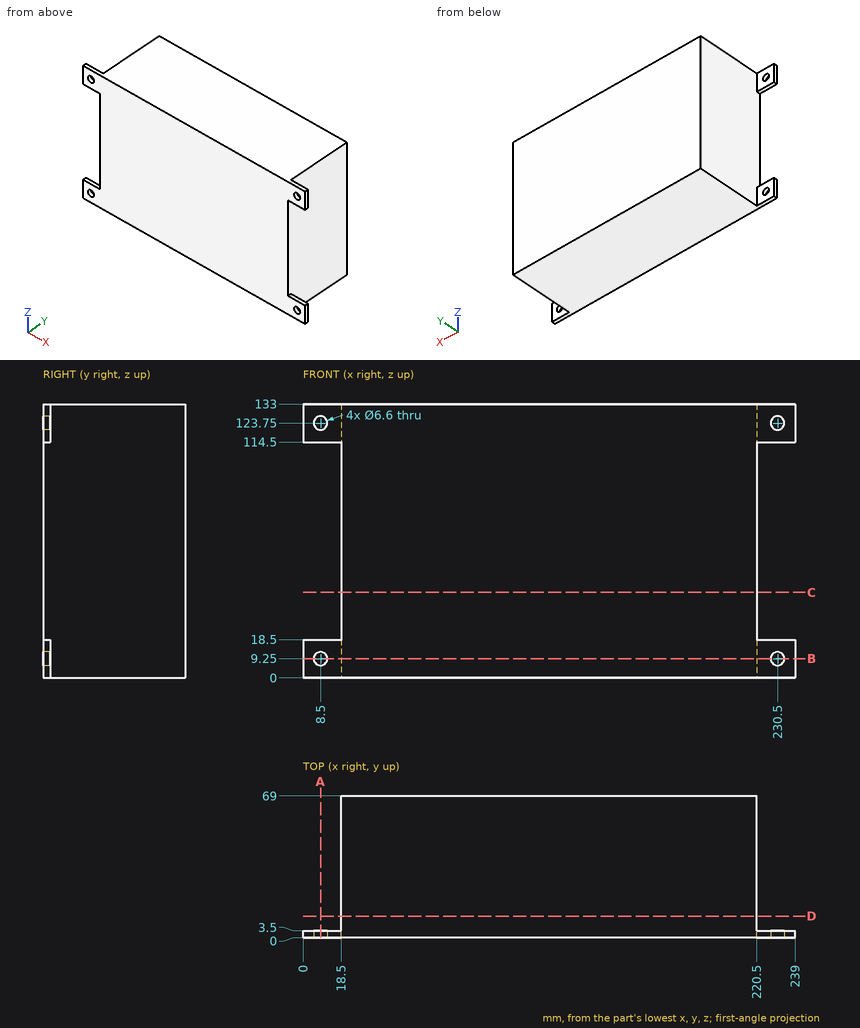
Design review of the part shown in the three views and the two pictorial views. Dimensions are in mm from the part's minimum x, y and z. Round coordinates to 2 decimals unless told otherwise and drop trailing zeros. Order: outer loops, then holes, each group sorted by start corner. A loop starts at its lowest first (then second) coordinate and runs counter-clockwise, first axis right, second up.
Q1. We need section B-B, the plane z = 9.25. Give the boundary of the cut face in (x, y), plus the area to 3 significant figures.
Findings below:
outline: (0, 0) - (5.2, 0) - (5.2, 3.5) - (0, 3.5) - close; (11.8, 0) - (227.2, 0) - (227.2, 3.5) - (220.5, 3.5) - (220.5, 69) - (18.5, 69) - (18.5, 3.5) - (11.8, 3.5) - close; (233.8, 0) - (239, 0) - (239, 3.5) - (233.8, 3.5) - close
area: 14,000 mm2
Q2. Insertion check: P1, Ø5, axis at x = 150.5, z = 67.5, coming from the -Y side; P2, Ø5, axis at y = 14.5, z = 116.5, coming from the -X side; P3, Ø5, axis at y = 43, z = 89.5, coming from the +X side; P4, Ø20.5, axis at x = 5, z = 122.5, coming from the +Y side. Each pin has a flat end and moves straight along its axis. Give the tip position at first contact, or say it passes through.
Findings below:
P1: stops at y = 0
P2: stops at x = 18.5
P3: stops at x = 220.5
P4: stops at y = 3.5
Q3. Wall thickness on line 1 (Z direction, x = 8.5, y = 2.45); line 2 (X direction, y = 2.55, z = 123.75); line 3 (X direction, y = 41.5, z = 108.5): over which ranges is each line inside the solid? List them lowest first.
Findings below:
line 1: z = 0 to 5.95, 12.55 to 18.5, 114.5 to 120.45, 127.05 to 133
line 2: x = 0 to 5.2, 11.8 to 227.2, 233.8 to 239
line 3: x = 18.5 to 220.5
Q4. We need section D-D, the plane y = 10.5. Give the boundary of the cut face in (x, z).
Findings below:
outline: (18.5, 0) - (220.5, 0) - (220.5, 133) - (18.5, 133) - close
Q5. We need section A-A, the plane x = 8.5. Give the boundary of the cut face in (y, z).
Findings below:
outline: (0, 0) - (3.5, 0) - (3.5, 5.95) - (0, 5.95) - close; (0, 12.55) - (3.5, 12.55) - (3.5, 18.5) - (0, 18.5) - close; (0, 114.5) - (3.5, 114.5) - (3.5, 120.45) - (0, 120.45) - close; (0, 127.05) - (3.5, 127.05) - (3.5, 133) - (0, 133) - close
Q6. We need section C-C, the plane z = 41.5. Give the boundary of the cut face in (x, y), plus the area to 3 significant figures.
Findings below:
outline: (18.5, 0) - (220.5, 0) - (220.5, 69) - (18.5, 69) - close
area: 13,900 mm2
